```python
from build123d import *

# Parameters (mm, degrees)
F1_DEPTH  = 24.3586
F2_R      = 38.735
F3_DEPTH  = 12.7
F4_R      = 32.893
F5_DEPTH  = 25.1714
F7_DEPTH  = 100.584
F11_ANGLE = 180
F12_ANGLE = 180
F13_DEPTH = 25.4
F14_R     = 29.21
F15_DEPTH = 12.7
F16_R     = 22.86
F16_R_2   = 15.24
F17_DEPTH = 101.6


with BuildPart() as f1:
    # F0 (on Front) → F1 (new body)
    with BuildSketch(Plane.XZ):
        with BuildLine():
            Line((-38.8343915367, 56.765781418), (-44.7878576566, 5.1676911222))
            ThreePointArc((-44.7878576566, 5.1676911222), (-45.0106531137, 2.588113459), (-45.085, 0))
            Line((-45.085, 0), (-75.4296230072, -31.7507315176))
            ThreePointArc((-75.4296230072, -31.7507315176), (-78.8758954242, -39.1705564298), (-77.0821164183, -47.1525957793))
            ThreePointArc((-77.0821164183, -47.1525957793), (0, -90.3605), (77.0821164183, -47.1525957793))
            ThreePointArc((77.0821164183, -47.1525957793), (78.8758954242, -39.1705564298), (75.4296230072, -31.7507315176))
            Line((75.4296230072, -31.7507315176), (45.085, 0))
            ThreePointArc((45.085, 0), (45.0106531137, 2.588113459), (44.7878576566, 5.1676911222))
            Line((44.7878576566, 5.1676911222), (38.8343915367, 56.765781418))
            ThreePointArc((38.8343915367, 56.765781418), (0, 90.3605), (-38.8343915367, 56.765781418))
        make_face()
    extrude(amount=F1_DEPTH)

    # F2 (on face) → F3 (join)
    with BuildSketch(Plane.XZ.offset(24.3586)):
        Circle(F2_R)
    extrude(amount=F3_DEPTH)

    # F4 (on face) → F5 (join)
    with BuildSketch(Plane(origin=(0, 0, 0), x_dir=(-1, 0, 0), z_dir=(0, 1, 0))):
        with Locations((0, 51.1175)):
            Circle(F4_R)
    extrude(amount=F5_DEPTH)

    # F6 (on Right) → F7 (cut, symmetric)
    with BuildSketch(Plane.YZ):
        Polygon((-9.2324605212, 94.8371365666), (-19.2786, 95.6272567787), (-70.8548203111, 97.9044958949), (-24.3586, 40.005), align=None)
    extrude(amount=F7_DEPTH, both=True, mode=Mode.SUBTRACT)

    # F8: F1 across face


with BuildPart() as f1_1:
    add(f1.part)
    add(f1.part.mirror(Plane(origin=(0, 25.1714, 51.1175), x_dir=(-1, 0, 0), z_dir=(0, 1, 0))))


with BuildPart() as f9_1:
    # F9: instance of F1
    add(f1_1.part.mirror(Plane(origin=(0, 87.4014, 0), x_dir=(-1, 0, 0), z_dir=(0, 1, 0))))


with BuildPart() as f10_1:
    # F10: instance of F9_1
    add(f9_1.part.mirror(Plane(origin=(0, 211.8614, 0), x_dir=(-1, 0, 0), z_dir=(0, 1, 0))))


with BuildPart() as f10_2:
    # F10: instance of F1
    add(f1_1.part.mirror(Plane(origin=(0, 211.8614, 0), x_dir=(-1, 0, 0), z_dir=(0, 1, 0))))


with BuildPart() as f9_1_1:
    # F11: moved
    add(f9_1.part.rotate(Axis((0, -37.0586, 0), (0, -1, 0)), F11_ANGLE))


with BuildPart() as f10_2_1:
    # F12: moved
    add(f10_2.part.rotate(Axis((0, -37.0586, 0), (0, -1, 0)), F12_ANGLE))


with BuildPart() as f1_2:
    add(f1_1.part)

    # F13 (add): a face of the model
    f13_faces = [f1_2.faces().sort_by_distance(p)[0] for p in [
        (0, -37.0586, 0),
    ]]
    extrude(f13_faces, amount=F13_DEPTH)

    # F14 (on face) → F15 (join)
    with BuildSketch(Plane.XZ.offset(62.4586)):
        Circle(F14_R)
    extrude(amount=F15_DEPTH)

    add(f9_1_1.part)  # F17 merges F9_1

    add(f10_1.part)  # F17 merges F10_1

    add(f10_2_1.part)  # F17 merges F10_2
    # F16 (on face) → F17 (join)
    with BuildSketch(Plane.XZ.offset(75.1586)):
        Circle(F16_R)
        Circle(F16_R_2, mode=Mode.SUBTRACT)
    extrude(amount=F17_DEPTH)


solid = f1_2.part
```
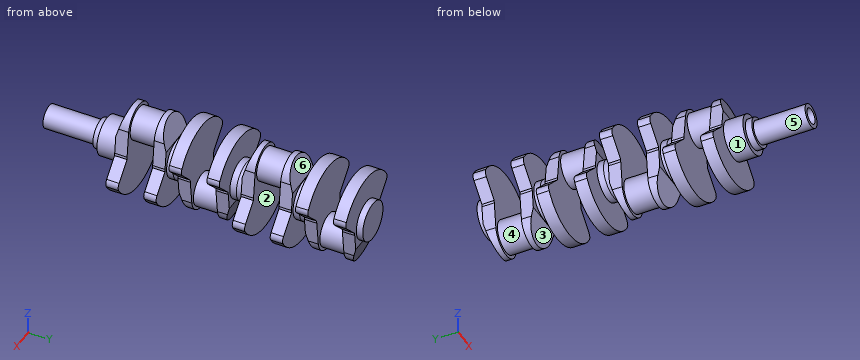
Geometry check sheet. Reference: the model listing, model coordinates, mm. Face numbers are marked on the shaded views. A direction names the side the tool comes from. Coordinates: 2 decimals unless noted, no trailing zeros. Write each loop counter-clockwise with the first axis right and the second up, starting at its lowest first coordinate (ties: lowest second). Pieces come first, ordered by that corner, then holes. Notation, with made-up numbers: M 51,42.5 L 64,42.5 A23 cw 64,66.5 Z; hole C 45,-26 d3. An arc over 180 degrees is marked long. Use one line per item in the form item = value. Start each with the question number.
1) Go/stop test with flat-tipped pins: pin 1 Ø3 at (y, z) = (285.5, 59.5) entering from +X; pin 2 Ø15 at (x, z) = (2, -6.5) entering from -Y; pin 3 Ø3 at (y, z) = (-94, 4.5) entering from +X. Record where each tip stops, or that it passes through.
2) Set-up check for the marked faces 3, 4, 5 and 6: record each of +Z, -Z, +X, -X, +Y, -Y from which the full face is reachable in a straight line by a thin tool's end or side.
3) Section check B-B on y = 282. Enter the section's corners in (x, z).
4) Thickness scan on probe 1 along Y at (x, z) = (53, -54.5); probe 2 along Y at (x, z) = (26, -40); probe 3 along Y at (x, z) = (-51.5, 24.5). Record the ranges inside material, lowest first. Write a range as from..to.
5) Release check for a two-part mould opening along Y. For the marked faces 1 and 2 record: pulls with the +Y half, pulls with the -Y half, needs draft (parallel to the pull), parting line crosses it, or undercut.
6) Section check A-A on x = -53.5. State how many separate pieces and enclosed holes the cut face has, and give its area (3 significant figures).
Responses:
q1.pin_1 = 32.16
q1.pin_2 = -75.16
q1.pin_3 = 22.66
q2.face_3 = -Z, +X, -X
q2.face_4 = none
q2.face_5 = -Y
q2.face_6 = +Z, +X, -X
q3.outline = C 0,51.12 d65.79
q4.probe_1 = -24.36..0, 50.34..74.7, 224.56..248.92, 299.26..323.62
q4.probe_2 = -24.36..0, 50.34..74.7, 100.1..199.16, 224.56..248.92, 299.26..323.62, 349.02..448.08
q4.probe_3 = 100.1..124.46, 174.8..199.16, 349.02..373.38, 423.72..448.08
q5.face_1 = needs draft
q5.face_2 = undercut
q6.separate_pieces = 8
q6.enclosed_holes = 0
q6.area = 12,500 mm2
